from build123d import *

# Parameters (mm, degrees)
SKETCH1_W               = 60
SKETCH1_H               = 65
SKETCH1_W_2             = 55
SKETCH1_H_2             = 60
BOSS_EXTRUDE1_DEPTH     = 40
SKETCH2_W               = 60
SKETCH2_H               = 65
BOSS_EXTRUDE2_DEPTH     = 2.5
BOSS_EXTRUDE3_DEPTH     = 65
CUT_EXTRUDE1_REACH      = 83.03
CUT_EXTRUDE2_DEPTH      = 84.873058845
CUT_EXTRUDE2_DEPTH_BACK = 84.873058845
SKETCH5_W               = 60
SKETCH5_H               = 41
SNAP_START              = -17.466738465
SNAP_HOOK1_DEPTH        = 0.923076923
SNAP_START_2            = -1.762465991
SNAP_HOOK1_2_DEPTH      = 3.524931982
SNAP_START_3            = -1.989936516
SNAP_HOOK1_3_DEPTH      = 3.979873032
SNAP_START_4            = -19
SNAP_HOOK1_4_DEPTH      = 5
CUT_EXTRUDE3_DEPTH      = 73.867619695
CUT_EXTRUDE3_DEPTH_BACK = 73.867619695
SKETCH6_W               = 60.42921797
SKETCH6_H               = 2.598338556


with BuildPart() as part:
    # Sketch1 → Boss-Extrude1 (new body)
    with BuildSketch(Plane(origin=(0, 0, 0), x_dir=(1, 0, 0), z_dir=(0, 1, 0))):
        Rectangle(SKETCH1_W, SKETCH1_H)
        Rectangle(SKETCH1_W_2, SKETCH1_H_2, mode=Mode.SUBTRACT)
    extrude(amount=BOSS_EXTRUDE1_DEPTH)

    # Sketch2 → Boss-Extrude2 (add)
    with BuildSketch(Plane(origin=(0, 40, 0), x_dir=(1, 0, 0), z_dir=(0, 1, 0))):
        Rectangle(SKETCH2_W, SKETCH2_H)
    extrude(amount=BOSS_EXTRUDE2_DEPTH)

    # Sketch3 → Boss-Extrude3 (add)
    with BuildSketch(Plane(origin=(0, 0, -32.5), x_dir=(-1, 0, 0), z_dir=(0, 0, -1))):
        Polygon((-30, 42.5), (-28.8, 43.7), (-27.6, 42.5), (-26.4, 43.7), (-25.2, 42.5), (-24, 43.7), (-22.8, 42.5), (-21.6, 43.7), (-20.4, 42.5), (-19.2, 43.7), (-18, 42.5), (-16.8, 43.7), (-15.6, 42.5), (-14.4, 43.7), (-13.2, 42.5), (-12, 43.7), (-10.8, 42.5), (-9.6, 43.7), (-8.4, 42.5), (-7.2, 43.7), (-6, 42.5), (-4.8, 43.7), (-3.6, 42.5), (-2.4, 43.7), (-1.2, 42.5), (0, 43.7), (1.2, 42.5), (2.4, 43.7), (3.6, 42.5), (4.8, 43.7), (6, 42.5), (7.2, 43.7), (8.4, 42.5), (9.6, 43.7), (10.8, 42.5), (12, 43.7), (13.2, 42.5), (14.4, 43.7), (15.6, 42.5), (16.8, 43.7), (18, 42.5), (19.2, 43.7), (20.4, 42.5), (21.6, 43.7), (22.8, 42.5), (24, 43.7), (25.2, 42.5), (26.4, 43.7), (27.6, 42.5), (28.8, 43.7), (30, 42.5), (30, 42.170064374), (-30, 42.170064374), align=None)
    extrude(amount=-BOSS_EXTRUDE3_DEPTH)

    # Cut-Extrude1: up to this face of the body (flat: up to its plane)
    cut_extrude1_end = Plane(part.part.faces().sort_by_distance((30, 21.25, 0))[0])
    # Sketch4 → Cut-Extrude1 (cut, up to the picked face)
    with BuildSketch(Plane.ZY.offset(30), mode=Mode.PRIVATE) as cut_extrude1_sk1:
        with BuildLine():
            Line((-32.5, 42.5), (-32.5, 43.7))
            Line((-32.5, 43.7), (-31.3, 43.7))
            ThreePointArc((-31.3, 43.7), (-32.148528137, 43.348528137), (-32.5, 42.5))
        make_face()
    cut_extrude1_tool1 = split(extrude(cut_extrude1_sk1.sketch, amount=-CUT_EXTRUDE1_REACH, mode=Mode.PRIVATE), bisect_by=cut_extrude1_end, keep=Keep.BOTH, mode=Mode.PRIVATE)
    cut_extrude1 = cut_extrude1_tool1.solids().sort_by(Axis((-30, 43.431958, -32.231958), (1, 0, 0)))[0]
    add(cut_extrude1, mode=Mode.SUBTRACT)

    # Mirror1: Cut-Extrude1 across plane
    add(cut_extrude1.mirror(Plane.XY), mode=Mode.SUBTRACT)

    # Sketch5 → Cut-Extrude2 (cut, two sides: drawn at the far end of the back side and taken through both)
    with BuildSketch(Plane.XY.offset(32.5).offset(-CUT_EXTRUDE2_DEPTH_BACK)):
        with Locations((0, 20.5)):
            Rectangle(SKETCH5_W, SKETCH5_H)
    extrude(amount=CUT_EXTRUDE2_DEPTH + CUT_EXTRUDE2_DEPTH_BACK, mode=Mode.SUBTRACT)

    # Snap Hook1: read off the stored shape, not the designer's step
    # Snap Hook1 outline → Snap Hook1 (add)
    with BuildSketch(Plane.XY.offset(SNAP_START)):
        Polygon((-1.5, 35.4), (1.5, 35.4), (1.989936516, 41), (-1.989936516, 41), align=None)
    snap_hook1 = extrude(amount=SNAP_HOOK1_DEPTH)

    # Snap Hook1 2 outline → Snap Hook1 2 (add)
    with BuildSketch(Plane.YZ.offset(SNAP_START_2)):
        Polygon((38.4, -17.466738465), (35.4, -17.466738465), (37.9, -18.466738465), (38.4, -18.466738465), align=None)
        Polygon((35.4, -16.543661542), (41, -16.543661542), (41, -15.466738465), align=None)
    snap_hook1_2 = extrude(amount=SNAP_HOOK1_2_DEPTH)

    # Snap Hook1 3 outline → Snap Hook1 3 (add)
    with BuildSketch(Plane.YZ.offset(SNAP_START_3)):
        Polygon((35.4, -16.543661542), (41, -16.543661542), (41, -15.466738465), align=None)
    snap_hook1_3 = extrude(amount=SNAP_HOOK1_3_DEPTH)

    # Snap Hook1 4 outline → Snap Hook1 4 (cut)
    with BuildSketch(Plane.XY.offset(SNAP_START_4)):
        Polygon((-1.989936516, 41), (-1.989936516, 34), (-1.377515871, 34), align=None)
        Polygon((1.377515871, 34), (1.989936516, 34), (1.989936516, 41), align=None)
    snap_hook1_4 = extrude(amount=SNAP_HOOK1_4_DEPTH, mode=Mode.SUBTRACT)

    # Mirror2: Snap Hook1, Snap Hook1 2, Snap Hook1 3, Snap Hook1 4 across plane
    add(snap_hook1.mirror(Plane.XY))
    add(snap_hook1_2.mirror(Plane.XY))
    add(snap_hook1_3.mirror(Plane.XY))
    add(snap_hook1_4.mirror(Plane.XY), mode=Mode.SUBTRACT)

    # Sketch6 → Cut-Extrude3 (cut, two sides: drawn at the far end of the back side and taken through both)
    with BuildSketch(Plane(origin=(0, 0, -17.5), x_dir=(-1, 0, 0), z_dir=(0, 0, -1)).offset(-CUT_EXTRUDE3_DEPTH_BACK)):
        with Locations((0.214608985, 43.799169278)):
            Rectangle(SKETCH6_W, SKETCH6_H)
    extrude(amount=CUT_EXTRUDE3_DEPTH + CUT_EXTRUDE3_DEPTH_BACK, mode=Mode.SUBTRACT)


solid = part.part
Design review of the part built by this model. Coordinates are the model's own, in mm. A direction names the side the tool comes from. Round coordinates to 2 decimals unless told otherwise and drop trailing zeros. Write each loop counter-clockwise with the first axis right and the second up, starting at its lowest first coordinate (ties: lowest second). Pieces come first, ordered by that corner, then holes. Notation, with made-up numbers: (19, -15) -> (48, -15) arc R31 cw to (48, 24) -> close; hole circle Ø4 at (45.5, 61). An arc over 180 degrees is marked (long way). One line per question, with ' | ' between items.
(1) Wall thickness on line 1 (Y direction, x = -26.5, z = 9); line 2 (Z direction, x = 1, y = 35.5); line 3 (X direction, y = 40.5, z = -17): over which ranges is each line inside the solid? List them lowest first. Write a range as [from, to].
Result sheet:
line 1: [41, 42.5] | line 2: [-17.51, -16.52], [16.52, 17.51] | line 3: [-1.95, 1.95]
(2) Draft analysis for pull direction Z (two halves, no side actions). For faces 6 (the flat face through (-0.02, 36.63, -17.96)), 7 (the flat face through (-0.028, 38.239, -15.998)), 8 (the flat face through (30, 42, 0)), state which applies: released by +Z, released by -Z, zero draft, split by the parting line, or undercut.
Result sheet:
face 6: released by -Z | face 7: undercut | face 8: zero draft
(3) Insertion check: P1, Ø0.8, axis at x = 0.5, y = 40, coming from the +Z side; P2, Ø0.6, axis at x = 0, y = 38, coming from the +Z side; P3, Ø0.8, axis at x = 0.5, y = 40, coming from the -Z side; P4, Ø4, axis at y = 38, z = 5, coming from the -X side. Each pin has a flat end and moves straight along its axis. Give the tip position at first contact, or say it passes through.
Result sheet:
P1: z = 17.47 | P2: z = 18.47 | P3: z = -17.47 | P4: through
(4) Take a section at B-B, the plane x = -16. State the section outline as (y, z) points, and give its area (3 significant figures).
Result sheet:
outline: (41, -32.5) -> (42.5, -32.5) -> (42.5, 32.5) -> (41, 32.5) -> close | area: 97.5 mm2
(5) Take a section at A-A, the plane y = 37. State the section outline as (x, z) points.
Result sheet:
outline: (-1.64, -18.11) -> (1.64, -18.11) -> (1.64, -16.24) -> (-1.64, -16.24) -> close; (-1.64, 16.24) -> (1.64, 16.24) -> (1.64, 18.11) -> (-1.64, 18.11) -> close
(6) Take a section at C-C, the plane z = -24. State the section outline as (x, y) points, and give its area (3 significant figures).
Result sheet:
outline: (-30, 41) -> (30, 41) -> (30, 42.5) -> (-30, 42.5) -> close | area: 90.0 mm2
(7) Machinability: for faces 1 (the flat face through (-0.028, 38.239, 15.998)), 2 (the flat face through (0, 40, -17.467)), 3 (the flat face through (-1.75, 38.24, 16.99)), 4 (the flat face through (0, 42.5, 0)), 5 (the flat face through (0, 40, 17.467)), which of the approach directions +Z, -Z, +X, -X, +Y, -Y give a long, thin tool a straight path to every point of the face, cutting with its end or side? Answer none if there is none.
Result sheet:
face 1: +X, -X, -Y | face 2: -Z, +X, -X | face 3: +Z, -Z, -X, -Y | face 4: +Z, -Z, +X, -X, +Y | face 5: +Z, +X, -X
